from build123d import *

# Parameters (mm, degrees)
F1_DEPTH = 10
F2_R     = 3
F3_DEPTH = 8


with BuildPart() as f1:
    # F0 (on Front) → F1 (new body)
    with BuildSketch(Plane.XZ):
        with BuildLine():
            Line((34.3, 26.65), (-34.3, 26.65))
            Line((-34.3, 26.65), (-34.3, 24.05))
            Line((-34.3, 24.05), (-31.8, 24.05))
            Line((-31.8, 24.05), (17.5, 24.05))
            ThreePointArc((17.5, 24.05), (19, 25.55), (20.5, 24.05))
            ThreePointArc((20.5, 24.05), (20.06066, 22.98934), (19, 22.55))
            Line((19, 22.55), (19, -23.401669))
            ThreePointArc((19, -23.401669), (20.687298, -22.700862), (21.8, -24.15))
            Line((21.8, -24.15), (34.3, -24.15))
            Line((34.3, -24.15), (34.3, 26.65))
        make_face()
        with BuildLine():
            ThreePointArc((-30.3, -19.05), (-30.73934, -17.98934), (-31.8, -17.55))
            ThreePointArc((-31.8, -17.55), (-32.86066, -20.11066), (-30.3, -19.05))
        make_face()
        with BuildLine():
            Line((-31.8, 24.05), (-34.3, 24.05))
            Line((-34.3, 24.05), (-34.3, -26.65))
            Line((-34.3, -26.65), (34.3, -26.65))
            Line((34.3, -26.65), (34.3, -24.15))
            Line((34.3, -24.15), (21.8, -24.15))
            ThreePointArc((21.8, -24.15), (19.912702, -25.599138), (19, -23.401669))
            Line((19, -23.401669), (19, 22.55))
            ThreePointArc((19, 22.55), (17.93934, 22.98934), (17.5, 24.05))
            Line((17.5, 24.05), (-31.8, 24.05))
        make_face()
        with BuildLine():
            ThreePointArc((-30.3, -19.05), (-32.86066, -20.11066), (-31.8, -17.55))
            ThreePointArc((-31.8, -17.55), (-30.73934, -17.98934), (-30.3, -19.05))
        make_face(mode=Mode.SUBTRACT)
        with BuildLine():
            ThreePointArc((-31.8, 7.35), (-33.3, 8.85), (-31.8, 10.35))
            ThreePointArc((-31.8, 10.35), (-30.73934, 9.91066), (-30.3, 8.85))
            ThreePointArc((-30.3, 8.85), (-30.73934, 7.78934), (-31.8, 7.35))
        make_face(mode=Mode.SUBTRACT)
    extrude(amount=F1_DEPTH)

    # F2 (on face) → F3 (cut)
    with BuildSketch(Plane(origin=(0, 0, 0), x_dir=(-1, 0, 0), z_dir=(0, 1, 0))):
        with Locations((-19, 24.05)):
            Circle(F2_R)
        with Locations((31.8, 8.85)):
            Circle(F2_R)
        with Locations((31.8, -19.05)):
            Circle(F2_R)
        with Locations((-20.3, -24.15)):
            Circle(F2_R)
    extrude(amount=-F3_DEPTH, mode=Mode.SUBTRACT)


solid = f1.part
Geometry: final body of the model. Coordinates: model frame, mm. A direction names the side the tool comes from. Give positions to 0.01 mm unless a question says otherwise; leave off trailing zeros. Loops run counter-clockwise (first coordinate to the right, second up) from the corner with the lowest first, then second, coordinate; pieces in that order, holes last. Notation, with made-up numbers: M 73.25,46.5 L 84.25,46.5 A22 ccw 84.25,58.5 Z; hole C 68,-3 d8. An arc over 180 degrees is marked long. Put each result on its own line as item: value. Start each with the question number.
1) Cut plane A-A (y = -6). Output: boundary loops of the cut face in (x, z), then the cut area to 3 significant figures.
2) Access query for faces 1 (the flat face through (19.7, -8, -22.6)), 2 (the flat face through (0, 0, 0)). Directions: +Z, -Z, +X, -X, +Y, -Y. A direction counts if a zero-diameter tool reaches every point of the face in a straight line with its end or side. Return the directions, or none.
3) Contact query for flat-ended pins moving along their axis: pin 1 (1.7 mm diameter, centred on x = 19, z = 23.5, fed in from +Y); pin 2 (3 mm diameter, centred on x = 20.5, z = -25, fed in from +Y). Output: stop coordinate, or through.
4) Pull-direction query (X, two-part tool) for faces 3 (the cylindrical face through (19.11, -3.944, 21.052)), 4 (the flat face through (-34.3, -5, 0)), 5 (the flat face through (0, -10, 0)); classes: pulls with the +X half, pulls with the -X half, needs draft (parallel to the pull), parting line crosses it, or undercut.
5) Ray query, line 1 along Z through (x, y) = (-31.8, -9.6); line 2 along Z through (x, y) = (-31.8, -3.75); line 3 along X through (y, z) = (-9.55, -24.15). Return the intervals inside material, ascending.
Verdict:
1. outline: M -34.3,-26.65 L 18.64,-26.65 A3 cw long 21.96,-26.65 L 34.3,-26.65 L 34.3,26.65 L 20.5,26.65 A3 cw long 17.5,26.65 L -34.3,26.65 L -34.3,10.51 A3 cw long -34.3,7.19 L -34.3,-17.39 A3 cw long -34.3,-20.71 Z
1. area: 3,550 mm2
2. face 1: +Y
2. face 2: +Z, -Z, +X, -X, +Y
3. pin 1: through
3. pin 2: y = -8
4. face 3: undercut
4. face 4: pulls with the -X half
4. face 5: needs draft
5. line 1: -26.65 to -20.55, -17.55 to 7.35, 10.35 to 26.65
5. line 2: -26.65 to -22.05, -16.05 to 5.85, 11.85 to 26.65
5. line 3: -34.3 to 18.8, 21.8 to 34.3
